```python
from build123d import *

# Parameters (mm, degrees)
F1_DEPTH   = 87
F4_D       = 3.3
F4_ON_F3_D = 3.3
F5_R       = 5


with BuildPart() as f1:
    # F0 (on Top) → F1 (new body)
    with BuildSketch(Plane.XY):
        with BuildLine():
            Line((26, 23), (26, 0))
            Line((26, 0), (30, 0))
            Line((30, 0), (30, 26))
            Line((30, 26), (29, 26))
            ThreePointArc((29, 26), (26.8786796564, 25.1213203436), (26, 23))
        make_face()
        with BuildLine():
            Line((26, 0), (3, 0))
            ThreePointArc((3, 0), (0.8786796564, -0.8786796564), (0, -3))
            Line((0, -3), (0, -4))
            Line((0, -4), (30, -4))
            Line((30, -4), (30, 0))
            Line((30, 0), (26, 0))
        make_face()
    extrude(amount=F1_DEPTH)

    # F4 (through all)
    with Locations(Plane(origin=(26, 0, 0), x_dir=(0, -1, 0), z_dir=(-1, 0, 0))):
        with Locations((-17.25, 10.875), (-17.25, 76.125), (-8.625, 43.5)):
            Hole(F4_D / 2)

    # F4 on F3 (through all)
    with Locations(Plane(origin=(0, 0, 0), x_dir=(-1, 0, 0), z_dir=(0, 1, 0))):
        with Locations((-8.75, 9.1315675527), (-17.375, 43.5), (-8.75, 76.125)):
            Hole(F4_ON_F3_D / 2)

    # F5
    f5_edges = [f1.edges().sort_by_distance(p)[0] for p in [
        (26, 0, 43.5),
    ]]
    fillet(f5_edges, radius=F5_R)


solid = f1.part
```
The listing builds one solid part. Answer for the finished solid, in the listing's coordinates (mm). A direction names the side the tool comes from. Coordinates: 2 decimals unless noted, no trailing zeros. Loops run counter-clockwise (first coordinate to the right, second up) from the corner with the lowest first, then second, coordinate; pieces in that order, holes last. Notation, with made-up numbers: (30.5, 10) - (51.5, 10) arc R23 ccw to (51.5, 46) - close; hole circle Ø8 at (70.5, 15.25). An arc over 180 degrees is marked (long way). Use a Markdown table: item, result. Add a question column.
1) The part is cut by section C-C, the plane z = 43.5. Give the vertices of the cut face in (x, y) (3 decimals).
2) Find the intervals of material crossed by line 1 (Z direction, x = 28.45, y = 17.25) (3 decimals); line 2 (Z direction, x = 8.75, y = -0.95) (3 decimals); line 3 (Z direction, x = 26.25, y = 8.5), in increasing order.
3) Given pin 1 (9 mm diameter, centred on y = 12.5, z = 33.5, fed in from -X); pin 2 (5.5 mm diameter, centred on x = 13, z = 46.5, fed in from +Y), each flat-ended and moving along its own axis, determine where each tip first touches the part or whether it passes through.
4) For faces 4 (the cylindrical face through (18.262, -2.028, 44.891)), 5 (the flat face through (12, 0, 43)), determine the directions among +Z, -Z, +X, -X, +Y, -Y from which every point of the face is accessible in a straight line to the end or side of a thin tool.
5) The part is cut by section B-B, the plane y = 17.25. Give the vertices of the cut face in (x, z) (3 decimals), and give its area (3 significant figures).
6) The part is cut by section A-A, the plane x = 8.75. Give the vertices of the cut face in (y, z) (3 decimals).
7) The mould has two halves that part along Z. Classify faces 1 (the flat face through (30, 11, 43)), 2 (the cylindrical face through (8.54, -2.03, 77.76)), 3 (the flat face through (23, 0, 0)): released by +Z, released by -Z, zero draft, split by the parting line, or undercut.
8) The part is cut by section D-D, the plane z = 65. Give the vertices of the cut face in (x, y), and give its area (3 significant figures).
Here are the results:
| question | item | result |
|---|---|---|
| 1 | outline | (0, -4) - (15.725, -4) - (15.725, 0) - (3, 0) arc R3 ccw to (0, -3) - close; (19.025, -4) - (30, -4) - (30, 6.975) - (26, 6.975) - (26, 5) arc R5 cw to (21, 0) - (19.025, 0) - close; (26, 10.275) - (30, 10.275) - (30, 26) - (29, 26) arc R3 ccw to (26, 23) - close |
| 2 | line 1 | z = 0 to 9.225, 12.525 to 74.475, 77.775 to 87 |
| 2 | line 2 | z = 0 to 7.482, 10.782 to 74.475, 77.775 to 87 |
| 2 | line 3 | z = 0 to 41.85, 45.15 to 87 |
| 3 | pin 1 | stops at x = 26 |
| 3 | pin 2 | stops at y = 0 |
| 4 | face 4 | +Y, -Y |
| 4 | face 5 | +Z, -Z, -X, +Y |
| 5 | outline | (26, 0) - (30, 0) - (30, 9.225) - (26, 9.225) - close; (26, 12.525) - (30, 12.525) - (30, 74.475) - (26, 74.475) - close; (26, 77.775) - (30, 77.775) - (30, 87) - (26, 87) - close |
| 5 | area | 322 mm^2 |
| 6 | outline | (-4, 0) - (0, 0) - (0, 7.482) - (-4, 7.482) - close; (-4, 10.782) - (0, 10.782) - (0, 74.475) - (-4, 74.475) - close; (-4, 77.775) - (0, 77.775) - (0, 87) - (-4, 87) - close |
| 7 | face 1 | zero draft |
| 7 | face 2 | undercut |
| 7 | face 3 | released by -Z |
| 8 | outline | (0, -4) - (30, -4) - (30, 26) - (29, 26) arc R3 ccw to (26, 23) - (26, 5) arc R5 cw to (21, 0) - (3, 0) arc R3 ccw to (0, -3) - close |
| 8 | area | 226 mm^2 |
